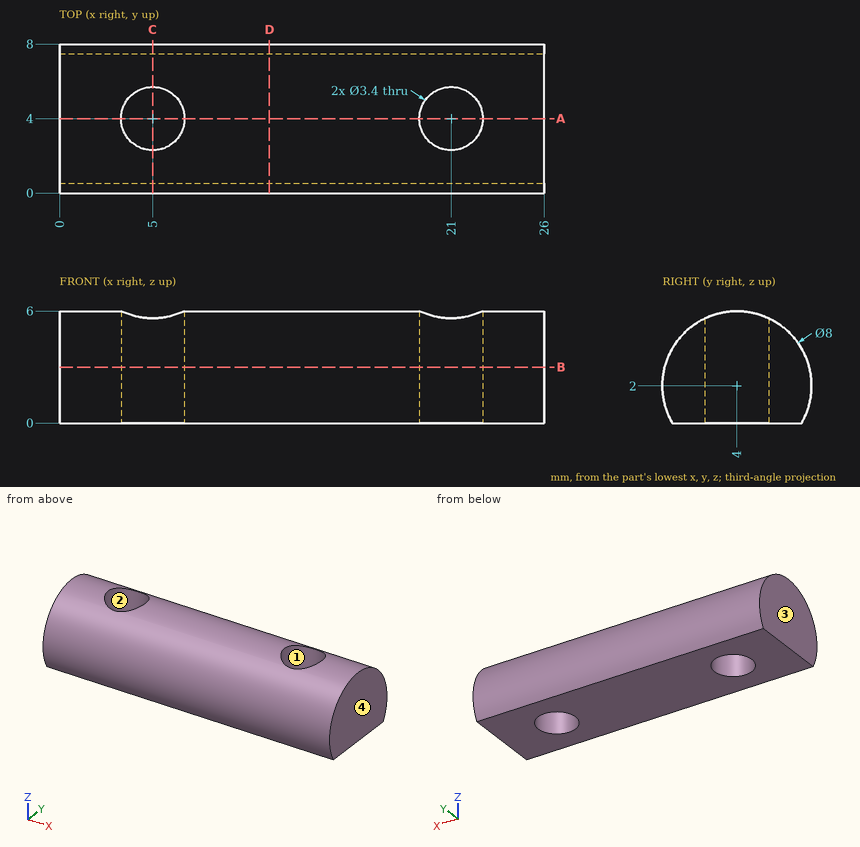
Source: three-view drawing plus pictorial views. Frame: mm from the lowest corner of the part. Round coordinates to 2 decimals unless told otherwise and drop trailing zeros. Write each loop counter-clockwise with the first axis right and the second up, starting at its lowest first coordinate (ties: lowest second). Pieces come first, ordered by that corner, then holes. Notation, with made-up numbers: M 54,-35 L 89,-35 A15 cw 89,-17 Z; hole C 52.25,-38 d7. An arc over 180 degrees is marked long. Write item = value, one per line.
Item 1: Section query A-A on y = 4. Return loops of the section in (x, z).
Findings:
outline = M 0,0 L 3.3,0 L 3.3,6 L 0,6 Z; M 6.7,0 L 19.3,0 L 19.3,6 L 6.7,6 Z; M 22.7,0 L 26,0 L 26,6 L 22.7,6 Z
Item 2: Material intervals for line 1 along X through (y, z) = (4, 4.75); line 2 along X through (y, z) = (5, 4); line 3 along Y through (x, z) = (4, 2), sorted ascending. Write a range as [from, to].
Findings:
line_1 = [0, 3.3], [6.7, 19.3], [22.7, 26]
line_2 = [0, 3.63], [6.37, 19.63], [22.37, 26]
line_3 = [0, 2.63], [5.37, 8]
Item 3: Section query C-C on x = 5. Return loops of the section in (y, z), then the cut area to 3 significant figures.
Findings:
outline = M 0.54,0 L 2.3,0 L 2.3,5.62 A4 ccw Z; M 5.7,0 L 7.46,0 A4 ccw 5.7,5.62 Z
area = 20.5 mm^2
Item 4: Section query B-B on z = 3. Return loops of the section in (x, y), then the cut area to 3 significant figures.
Findings:
outline = M 0,0.13 L 26,0.13 L 26,7.87 L 0,7.87 Z; hole C 5,4 d3.4; hole C 21,4 d3.4
area = 183 mm^2
Item 5: Section query D-D on x = 11.25. Return loops of the section in (y, z).
Findings:
outline = M 0.54,0 L 7.46,0 A4 ccw long Z
Item 6: Pull-direction query (X, two-part tool) for the marked faces 1, 2, 3 and 4; classes: pulls with the +X half, pulls with the -X half, needs draft (parallel to the pull), parting line crosses it, or undercut.
Findings:
face_1 = undercut
face_2 = undercut
face_3 = pulls with the -X half
face_4 = pulls with the +X half
